from build123d import *

# Parameters (mm, degrees)
SKETCH_1_R               = 15
EXTRUDE_1_DEPTH          = 265
CUT_EXTRUDE_1_DEPTH      = 266.847700761
CUT_EXTRUDE_1_DEPTH_BACK = 266.847700761
SKETCH_2_R               = 1.5
CUT_EXTRUDE_2_REACH      = 267.848
SKETCH_3_R               = 14


with BuildPart() as part:
    # 草圖1 → 填料-伸長1 (new body)
    with BuildSketch(Plane(origin=(0, 0, 0), x_dir=(1, 0, 0), z_dir=(0, 1, 0))):
        with Locations(Location((0, 0, 0), (0, 0, 270))):
            Circle(SKETCH_1_R)
    extrude(amount=EXTRUDE_1_DEPTH)

    # 草圖2 → 除料-伸長1 (cut, two sides: drawn at the far end of the back side and taken through both)
    with BuildSketch(Plane.XY.offset(-CUT_EXTRUDE_1_DEPTH_BACK)):
        with Locations((0, 255)):
            Circle(SKETCH_2_R)
        with Locations((0, 235)):
            Circle(SKETCH_2_R)
        with Locations((0, 10)):
            Circle(SKETCH_2_R)
        with Locations((0, 30)):
            Circle(SKETCH_2_R)
    extrude(amount=CUT_EXTRUDE_1_DEPTH + CUT_EXTRUDE_1_DEPTH_BACK, mode=Mode.SUBTRACT)

    # 草圖3 → 除料-伸長2 (cut, up to next)
    with BuildSketch(Plane(origin=(0, 265, 0), x_dir=(1, 0, 0), z_dir=(0, 1, 0)), mode=Mode.PRIVATE) as cut_extrude_2_sk1:
        with Locations(Location((0, 0, 0), (0, 0, 270))):
            Circle(SKETCH_3_R)
    cut_extrude_2_tool1 = extrude(cut_extrude_2_sk1.sketch, amount=-CUT_EXTRUDE_2_REACH, mode=Mode.PRIVATE) & part.part
    add(cut_extrude_2_tool1.solids().sort_by_distance((0, 265, 0))[0], mode=Mode.SUBTRACT)


solid = part.part
Input: part model. Units: mm. Frame: model coordinates. Give positions to 0.01 mm unless a question says otherwise; leave off trailing zeros. Order: outer loops, then holes, each group sorted by start corner. A loop starts at its lowest first (then second) coordinate and runs counter-clockwise, first axis right, second up. Notation, with made-up numbers: (76, -4.75) -> (135, -4.75) arc R25 cw to (135, 28.25) -> close; hole circle Ø4 at (-34.5, 50.25). An arc over 180 degrees is marked (long way). Use one line per item in the form item = value.
1) Mould query, pull axis Z, two halves, no side actions, for faces 1 (the cylindrical face through (-13.67, 134.35, -3.03)), 2 (the cylindrical face through (0.66, 130.645, -14.985)). Classes: pulls with the +Z half, pulls with the -Z half, needs draft (parallel to the pull), parting line crosses it, or undercut.
Response values:
face_1 = undercut
face_2 = parting line crosses it
2) Line query: probe 1 along Y at (x, z) = (0, 14.5); probe 2 along Z at (x, y) = (0, 72.5); probe 3 along Z at (x, y) = (10, 151.5). Output: solid intervals per line, ascending.
Response values:
probe_1 = 0 to 8.5, 11.5 to 28.5, 31.5 to 233.5, 236.5 to 253.5, 256.5 to 265
probe_2 = -15 to -14, 14 to 15
probe_3 = -11.18 to -9.8, 9.8 to 11.18
3) Section B-B, the plane y = 218. Return loops of the section in (x, z), and give its area (3 significant figures).
Response values:
outline = circle Ø30 at (0, 0); hole circle Ø28 at (0, 0)
area = 91.1 mm^2
4) First-contact query: pin 1 Ø10 at (y, z) = (197.5, 10.5) entering from +X; pin 2 Ø1 at (x, y) = (2.5, 88) entering from -Z; pin 3 Ø2.5 at (x, y) = (0, 30) entering from +Z; pin 4 Ø5 at (x, y) = (0, 235) entering from +Z. Flat tips, straight axial feed; report the tip coordinate or a pass-through.
Response values:
pin_1 = 13.96
pin_2 = -14.87
pin_3 = through
pin_4 = 15
5) Section A-A, the plane z = 0. Return loops of the section in (x, y).
Response values:
outline = (-15, 0) -> (-14, 0) -> (-14, 265) -> (-15, 265) -> close; (14, 0) -> (15, 0) -> (15, 265) -> (14, 265) -> close
6) Section C-C, the plane z = 10.5. Return loops of the section in (x, y).
Response values:
outline = (-10.71, 0) -> (-9.26, 0) -> (-9.26, 265) -> (-10.71, 265) -> close; (9.26, 0) -> (10.71, 0) -> (10.71, 265) -> (9.26, 265) -> close
